from build123d import *

# Parameters (mm, degrees)
EXTRUDE_1_DEPTH     = 3
SKETCH_2_OUTSIDE_W  = 13.724
SKETCH_2_OUTSIDE_H  = 8.024
CUT_EXTRUDE_1_DEPTH = 12
SKETCH_3_R          = 1
CUT_EXTRUDE_2_DEPTH = 12
FILLET_1_R          = 1
SKETCH_4_R          = 0.95
EXTRUDE_2_DEPTH     = 2
SKETCH_5_W          = 8
SKETCH_5_H          = 3
EXTRUDE_3_DEPTH     = 6
SKETCH_6_R          = 1
CUT_EXTRUDE_3_DEPTH = 12
CUT_EXTRUDE_4_DEPTH = 8
FILLET_2_R          = 1
SKETCH_11_W         = 8
SKETCH_11_H         = 3
EXTRUDE_4_DEPTH     = 2
SKETCH_12_W         = 4
SKETCH_12_H         = 4
CUT_EXTRUDE_5_DEPTH = 10


with BuildPart() as part:
    # 草图1 → 凸台-拉伸1 (new body)
    with BuildSketch(Plane(origin=(0, 0, 0), x_dir=(1, 0, 0), z_dir=(0, 1, 0))):
        Polygon((-6, 0), (6, 0), (6, -8.7), (4, -8.7), (4, -3), (-4, -3), (-4, -8.7), (-6, -8.7), align=None)
    extrude(amount=EXTRUDE_1_DEPTH)

    # 草图2 outside → 切除-拉伸1 (cut)
    with BuildSketch(Plane.ZY.offset(6)):
        with Locations((4.35, 1.5)):
            Rectangle(SKETCH_2_OUTSIDE_W, SKETCH_2_OUTSIDE_H)
        with BuildLine():
            Line((6.2, 3), (0, 3))
            Line((0, 3), (0, 0))
            Line((0, 0), (6.2, 0))
            ThreePointArc((6.2, 0), (7.7, 1.5), (6.2, 3))
        make_face(mode=Mode.SUBTRACT)
    extrude(amount=-CUT_EXTRUDE_1_DEPTH, mode=Mode.SUBTRACT)

    # 草图3 → 切除-拉伸2 (cut)
    with BuildSketch(Plane.ZY.offset(6)):
        with Locations((5.2, 1.5)):
            Circle(SKETCH_3_R)
    extrude(amount=-CUT_EXTRUDE_2_DEPTH, mode=Mode.SUBTRACT)

    # 圆角1
    fillet_1_edges = [part.edges().sort_by_distance(p)[0] for p in [
        (-6, 1.5, 0),
        (6, 1.5, 0),
    ]]
    fillet(fillet_1_edges, radius=FILLET_1_R)

    # 草图4 → 凸台-拉伸2 (add)
    with BuildSketch(Plane(origin=(0, 0, 0), x_dir=(-1, 0, 0), z_dir=(0, 0, -1))):
        with Locations(Location((0, 1.5, 0), (0, 0, 180))):
            Circle(SKETCH_4_R)
    extrude(amount=EXTRUDE_2_DEPTH)

    # 草图5 → 凸台-拉伸3 (add)
    with BuildSketch(Plane(origin=(0, 0, -2), x_dir=(-1, 0, 0), z_dir=(0, 0, -1))):
        with Locations((0, 1.5)):
            Rectangle(SKETCH_5_W, SKETCH_5_H)
    extrude(amount=EXTRUDE_3_DEPTH)

    # 草图6 → 切除-拉伸3 (cut)
    with BuildSketch(Plane(origin=(4, 0, 0), x_dir=(0, 0, -1), z_dir=(1, 0, 0))):
        with Locations(Location((6, 1.5, 0), (0, 0, 90))):
            Circle(SKETCH_6_R)
    extrude(amount=-CUT_EXTRUDE_3_DEPTH, mode=Mode.SUBTRACT)

    # 草图8 → 切除-拉伸4 (cut)
    with BuildSketch(Plane(origin=(0, 3, 0), x_dir=(1, 0, 0), z_dir=(0, 1, 0))):
        Polygon((-2, 10), (2, 8), (2, 3), (-2, 3), align=None)
    extrude(amount=-CUT_EXTRUDE_4_DEPTH, mode=Mode.SUBTRACT)

    # 圆角2
    fillet_2_edges = [part.edges().sort_by_distance(p)[0] for p in [
        (-3, 0, -8),
        (3, 0, -8),
    ]]
    fillet(fillet_2_edges, radius=FILLET_2_R)

    # 草图11 → 凸台-拉伸4 (add)
    with BuildSketch(Plane.XY.offset(-2)):
        with Locations((0, 1.5)):
            Rectangle(SKETCH_11_W, SKETCH_11_H)
    extrude(amount=EXTRUDE_4_DEPTH)

    # 草图12 → 切除-拉伸5 (cut)
    with BuildSketch(Plane(origin=(0, 3, 0), x_dir=(1, 0, 0), z_dir=(0, 1, 0))):
        with Locations((0, 1)):
            Rectangle(SKETCH_12_W, SKETCH_12_H)
    extrude(amount=-CUT_EXTRUDE_5_DEPTH, mode=Mode.SUBTRACT)


solid = part.part
The model under review builds one solid part; all positions refer to its coordinate system, in mm. A direction names the side the tool comes from. Give positions to 0.01 mm unless a question says otherwise; leave off trailing zeros. Order: outer loops, then holes, each group sorted by start corner. A loop starts at its lowest first (then second) coordinate and runs counter-clockwise, first axis right, second up. Notation, with made-up numbers: M 29.25,4 L 49.25,4 A13 cw 49.25,19 Z; hole C 66.25,10.5 d2. An arc over 180 degrees is marked long. Answer in a Markdown table with one row per item. Add a question column.
1. Add section B-B on z = -6. State the section outline as (x, y) points.
2. Add section A-A on z = -4.25. State the section outline as (x, y) points.
3. For pin 1 Ø1.5 at (y, z) = (1, -3.5) entering from -X; pin 2 Ø1 at (x, y) = (0, 1) entering from -Z; pin 3 Ø0.5 at (x, y) = (-4.5, 2) entering from -Z, all flat-tipped, find the tip position at first contact; note any pin that passes through.
4. Add section D-D on y = 2.05. Count the separate pieces of the cut face and the enclosed holes in it, plus the area to 3 significant figures.
5. Mouldability with a two-part tool opening along X and no side actions: class faces 1 (the flat face through (-2, 2, -3)), 2 (the cylindrical face through (5.699, 1.521, 0.285)), 3 (the flat face through (0, 0, 2)), 4 (the flat face through (0, 1, 3)) as released by +X, released by -X, zero draft, split by the parting line, or undercut.
6. Add section C-C on x = -2.5. State the section outline as (y, z) points, plus the area to 3 significant figures.
7. To check wall thickness, follow line 1 along X through (y, z) = (0.5, -0.5); line 2 along Y through (x, z) = (-4.8, 5.2); line 3 along Z through (x, y) = (2.9, 1.5). State the ranges of each line that lie inside material, in increasing order.
8. Machinability: for faces 5 (the cylindrical face through (-5.014, 1.117, 6.124)), 6 (the flat face through (4.5, 1.5, 0)), 7 (the flat face through (-4, 2, 4)), 8 (the flat face through (0, 2, 1)), which of the approach directions +Z, -Z, +X, -X, +Y, -Y give a long, thin tool a straight path to every point of the face, cutting with its end or side? Answer none if there is none.
The answers:
| question | item | result |
|---|---|---|
| 1 | outline | M -4,0 L -2,0 L -2,0.5 L -4,0.5 Z; M -4,2.5 L -2,2.5 L -2,3 L -4,3 Z; M 2,0 L 4,0 L 4,0.5 L 2,0.5 Z; M 2,2.5 L 4,2.5 L 4,3 L 2,3 Z |
| 2 | outline | M -4,0 L -2,0 L -2,3 L -4,3 Z; M 2,0 L 4,0 L 4,3 L 2,3 Z |
| 3 | pin 1 | x = -4 |
| 3 | pin 2 | z = 1 |
| 3 | pin 3 | z = 0 |
| 4 | separate pieces | 5 |
| 4 | enclosed holes | 0 |
| 4 | area | 68.6 mm2 |
| 5 | face 1 | undercut |
| 5 | face 2 | released by +X |
| 5 | face 3 | zero draft |
| 5 | face 4 | undercut |
| 6 | outline | M 0,-7 A1 ccw 1,-8 L 3,-8 L 3,3 L 0,3 Z; hole C 1.5,-6 d2 |
| 6 | area | 29.6 mm2 |
| 7 | line 1 | -4 to -2, 2 to 4 |
| 7 | line 2 | 0 to 0.5, 2.5 to 3 |
| 7 | line 3 | -8 to -7, -5 to 3 |
| 8 | face 5 | +X, -X |
| 8 | face 6 | -Z, +X, +Y, -Y |
| 8 | face 7 | +Z, +Y, -Y |
| 8 | face 8 | -Z, +Y, -Y |
